The listing builds one solid part. Answer for the finished solid, in the listing's coordinates (mm). A direction names the side the tool comes from. Round coordinates to 2 decimals unless told otherwise and drop trailing zeros. Write each loop counter-clockwise with the first axis right and the second up, starting at its lowest first coordinate (ties: lowest second). Pieces come first, ordered by that corner, then holes.
from build123d import *

# Parameters (mm, degrees)
SKETCH_1_W          = 46
SKETCH_1_H          = 21.3
EXTRUDE_1_DEPTH     = 2
SKETCH_2_R          = 8.25
CUT_EXTRUDE_1_DEPTH = 3
SKETCH_3_W          = 8
SKETCH_3_H          = 3
CUT_EXTRUDE_2_DEPTH = 3
SKETCH_4_W          = 5
SKETCH_4_H          = 4
CUT_EXTRUDE_3_DEPTH = 3
SKETCH_5_W          = 3
SKETCH_5_H          = 2
SKETCH_5_W_2        = 2
SKETCH_5_H_2        = 3
CUT_EXTRUDE_4_DEPTH = 1
HOLE_WIZARD_M3_1_D  = 3.4


with BuildPart() as part:
    # 草圖1 → 填料-伸長1 (new body)
    with BuildSketch(Plane.XY):
        Rectangle(SKETCH_1_W, SKETCH_1_H)
    extrude(amount=EXTRUDE_1_DEPTH)

    # 草圖2 → 除料-伸長1 (cut, through all)
    with BuildSketch(Plane.XY.offset(2)):
        with Locations((-12.7, 0)):
            Circle(SKETCH_2_R)
        with Locations((12.7, 0)):
            Circle(SKETCH_2_R)
    extrude(amount=-CUT_EXTRUDE_1_DEPTH, mode=Mode.SUBTRACT)

    # 草圖3 → 除料-伸長2 (cut, through all)
    with BuildSketch(Plane.XY.offset(2)):
        with Locations((0, 9.15)):
            Rectangle(SKETCH_3_W, SKETCH_3_H)
    extrude(amount=-CUT_EXTRUDE_2_DEPTH, mode=Mode.SUBTRACT)

    # 草圖4 → 除料-伸長3 (cut, through all)
    with BuildSketch(Plane.XY.offset(2)):
        with Locations((0, -5.5)):
            Rectangle(SKETCH_4_W, SKETCH_4_H)
    extrude(amount=-CUT_EXTRUDE_3_DEPTH, mode=Mode.SUBTRACT)

    # 草圖5 → 除料-伸長4 (cut)
    with BuildSketch(Plane.XY.offset(2)):
        with Locations((4, -6.5)):
            Rectangle(SKETCH_5_W, SKETCH_5_H)
        with Locations((-5.5, 8.65)):
            Rectangle(SKETCH_5_W_2, SKETCH_5_H_2)
        with Locations((5.5, 8.65)):
            Rectangle(SKETCH_5_W_2, SKETCH_5_H_2)
    extrude(amount=-CUT_EXTRUDE_4_DEPTH, mode=Mode.SUBTRACT)

    # M3 餘隙孔1 (through all)
    with Locations(Plane.XY.offset(2)):
        with Locations((0, 0), (20.35, 8.15), (-20.35, -8.15), (-20.35, 8.15), (20.35, -8.15)):
            Hole(HOLE_WIZARD_M3_1_D / 2)


solid = part.part
1. A tool of negligible diameter and unlimited length cuts with its end or side. For faces 1 (the face through (13, 10.65, 1)), 2 (the face through (-2.5, -6, 1)), 3 (the face through (-4, 9, 1)), 4 (the face through (5, 9, 1)), from which of +Z, -Z, +X, -X, +Y, -Y can it reach the whole face along a straight path? Write none if from no direction.
Geometry says:
face 1: +Z, -Z, +X, -X, +Y
face 2: +Z, -Z
face 3: +Z, -Z, +Y
face 4: +Z
2. Section B-B on x = 0 is taken. Determine the outline of the cut face in (y, z), plus the area to 3 significant figures.
Geometry says:
outline: (-10.65, 0) - (-7.5, 0) - (-7.5, 2) - (-10.65, 2) - close; (-3.5, 0) - (-1.7, 0) - (-1.7, 2) - (-3.5, 2) - close; (1.7, 0) - (7.65, 0) - (7.65, 2) - (1.7, 2) - close
area: 21.8 mm2
3. Section A-A on z = 0.3 is taken. Give the number of separate pieces and of enclosed holes in the cut face, plus the area to 3 significant figures.
Geometry says:
separate pieces: 1
enclosed holes: 8
area: 463 mm2
4. Section C-C on y = 0 is taken. Determine the outline of the cut face in (x, z).
Geometry says:
outline: (-23, 0) - (-20.95, 0) - (-20.95, 2) - (-23, 2) - close; (-4.45, 0) - (-1.7, 0) - (-1.7, 2) - (-4.45, 2) - close; (1.7, 0) - (4.45, 0) - (4.45, 2) - (1.7, 2) - close; (20.95, 0) - (23, 0) - (23, 2) - (20.95, 2) - close
5. Given pin 1 (0.6 mm diameter, centred on x = 3.5, z = 1, fed in from +Y), flat-ended and moving along its own axis, determine where the tip first touches the part or whether it passes through.
Geometry says:
pin 1: stops at y = 7.65
6. Straight lines are drawn through the part: line 1 along Y through (x, z) = (0, 0.5); line 2 along Y through (x, z) = (-12.7, 0.9); line 3 along X through (y, z) = (-1.75, 0.4). For each, find the intervals that lie inside material, in ascending order.
Geometry says:
line 1: y = -10.65 to -7.5, -3.5 to -1.7, 1.7 to 7.65
line 2: y = -10.65 to -8.25, 8.25 to 10.65
line 3: x = -23 to -20.76, -4.64 to 4.64, 20.76 to 23
7. Section D-D on y = -3 is taken. Determine the outline of the cut face in (x, z).
Geometry says:
outline: (-23, 0) - (-20.39, 0) - (-20.39, 2) - (-23, 2) - close; (-5.01, 0) - (5.01, 0) - (5.01, 2) - (-5.01, 2) - close; (20.39, 0) - (23, 0) - (23, 2) - (20.39, 2) - close
